from build123d import *

# Parameters (mm, degrees)
F1_DEPTH = 12.7


with BuildPart() as f1:
    # F0 (on Front) → F1 (new body)
    with BuildSketch(Plane.XZ):
        with BuildLine():
            Line((-24.285673, 10.139517), (-24.285673, 7.374194))
            Line((-24.285673, 7.374194), (-21.424013, 7.374194))
            Line((-21.424013, 7.374194), (-21.424013, 3.928539))
            ThreePointArc((-21.424013, 3.928539), (-21.779967, 0.066171), (-22.835836, -3.666084))
            Line((-22.835836, -3.666084), (-24.334839, -7.558548))
            Line((-24.334839, -7.558548), (-14.379678, -7.558548))
            Line((-14.379678, -7.558548), (-15.878681, -3.666084))
            ThreePointArc((-15.878681, -3.666084), (-16.93455, 0.066171), (-17.290504, 3.928539))
            Line((-17.290504, 3.928539), (-17.290504, 7.374194))
            Line((-17.290504, 7.374194), (-14.428843, 7.374194))
            Line((-14.428843, 7.374194), (-14.428843, 10.139517))
            Line((-14.428843, 10.139517), (-17.290504, 10.139517))
            Line((-17.290504, 10.139517), (-17.290504, 13.493787))
            Line((-17.290504, 13.493787), (-21.424013, 13.455031))
            Line((-21.424013, 13.455031), (-21.424013, 10.139517))
            Line((-21.424013, 10.139517), (-24.285673, 10.139517))
        make_face()
        Polygon((-20.272696, -2.44856), (-20.272696, 0), (-20.272696, 7.374194), (-20.272696, 8.660011), (-18.877488, 11.816652), (-18.722465, 7.374194), (-18.722465, 0), (-18.722465, -2.44856), (-17.933246, -2.44856), (-17.933246, -3.230711), (-18.722465, -3.230711), (-18.722465, -5.837881), (-20.272696, -5.837881), (-20.272696, -3.230711), (-21.127159, -3.230711), (-21.127159, -2.44856), align=None, mode=Mode.SUBTRACT)
    extrude(amount=F1_DEPTH)


solid = f1.part
Read the model definition and answer for the solid it produces. Units are mm, in the model's axes. A direction names the side the tool comes from. Give positions to 0.01 mm unless a question says otherwise; leave off trailing zeros. Write each loop counter-clockwise with the first axis right and the second up, starting at its lowest first coordinate (ties: lowest second). Pieces come first, ordered by that corner, then holes. Notation, with made-up numbers: M 14.5,27 L 44.5,27 A6 ccw 44.5,34 Z; hole C 77,-7.75 d10. An arc over 180 degrees is marked long. One line per item, written item: value. Start each with the question number.
(1) Find the intervals of material crossed by line 1 (X direction, y = -7.25, z = 6.75); line 2 (X direction, y = -12, z = -4.25); line 3 (Z direction, x = -19, y = -8.5), in increasing order.
(2) Determine the mould class of faces 1 (the flat face through (-18, 0, 3)), 2 (the flat face through (-20.273, -6, 3)), 3 (the cylindrical face through (-16.925, -6.261, 0.013)) for opening direction X: pulls with the +X half, pulls with the -X half, needs draft (parallel to the pull), parting line crosses it, or undercut.
(3) Flat-ended cylindrical pins translate along their axes: pin 1 Ø2.5 at (x, y) = (-16, -4) entering from +Z; pin 2 Ø1 at (x, y) = (-21.5, -11) entering from +Z; pin 3 Ø1 at (y, z) = (-2.5, -1.5) entering from +X. Find the tip coordinate at first contact, or state that the pin passes through.
(4) Find section C-C (x = -20.75). Determine the outline of the cut face in (y, z), plus the area to 3 significant figures.
(5) Find section B-B (z = 4.5). Determine the outline of the cut face in (x, y).
(6) A tool of negligible diameter and unlimited length cuts with its end or side. For faces 4 (the flat face through (-21.424, -6, 6)), 5 (the flat face through (-19, -6, -5.838)), 6 (the flat face through (-16, -6, 7.374)), from which of +Z, -Z, +X, -X, +Y, -Y can it reach the whole face along a straight path? Write none if from no direction.
Results below:
1. line 1: x = -21.42 to -20.27, -18.72 to -17.29
1. line 2: x = -23.06 to -20.27, -18.72 to -15.65
1. line 3: z = -7.56 to -5.84, 11.54 to 13.48
2. face 1: needs draft
2. face 2: undercut
2. face 3: pulls with the +X half
3. pin 1: stops at z = 10.14
3. pin 2: stops at z = 13.46
3. pin 3: stops at x = -16.44
4. outline: M -12.7,-7.56 L 0,-7.56 L 0,-3.23 L -12.7,-3.23 Z; M -12.7,-2.45 L 0,-2.45 L 0,13.46 L -12.7,13.46 Z
4. area: 257 mm^2
5. outline: M -21.42,-12.7 L -20.27,-12.7 L -20.27,0 L -21.42,0 Z; M -18.72,-12.7 L -17.29,-12.7 L -17.29,0 L -18.72,0 Z
6. face 4: -X, +Y, -Y
6. face 5: +Y, -Y
6. face 6: +X, +Y, -Y
